from build123d import *

# Parameters (mm, degrees)
F0_R     = 136.525
F0_R_2   = 79.375
F1_DEPTH = 50.8
F2_R     = 31.75
F4_R     = 19.05
F5_DEPTH = 38.1


# Not quite as in the source:
# - a fillet or chamfer that OpenCascade refuses, or shapes differently, is made with other operations: its cross-section is extruded or revolved along the edge and cut away or added


with BuildPart() as f1:
    # F0 (on Top) → F1 (new body)
    with BuildSketch(Plane.XY):
        with Locations((0, 2.0348737297)):
            Circle(F0_R)
        with Locations((0, 2.0348737297)):
            Circle(F0_R_2, mode=Mode.SUBTRACT)
    extrude(amount=F1_DEPTH)

    # F2
    f2_edges = [f1.edges().sort_by_distance(p)[0] for p in [
        (-136.525, 2.034874, 0),
    ]]
    fillet(f2_edges, radius=F2_R)

    # F3: fillet of radius 31.75 on 1 edges, made by hand

    # F3_s1 → F3_t2 (revolve, cut)
    with BuildSketch(Plane.XZ.offset(-2.0348737297)):
        with BuildLine():
            ThreePointArc((104.775, 0), (86.5315557516, 11.0280565913), (79.375, 31.1085197333))
            Line((79.375, 31.1085197333), (79.375, 0))
            Line((79.375, 0), (104.775, 0))
        make_face()
    revolve(axis=Axis((0, 2.0348737297, 0), (0, 0, 1)), mode=Mode.SUBTRACT)

    # F4 (on face) → F5 (cut)
    with BuildSketch(Plane.XY.offset(50.8)):
        with BuildLine():
            ThreePointArc((-83.5406207988, -89.6430518351), (-63.4036145785, -91.8975231455), (-52.6271930456, -74.7379660606))
            ThreePointArc((-52.6271930456, -74.7379660606), (-54.2244900151, -67.1021519632), (-58.7485218572, -60.74682739))
            ThreePointArc((-58.7485218572, -60.74682739), (-86.1351193385, -62.3334964102), (-83.5406207988, -89.6430518351))
        make_face()
        with BuildLine():
            ThreePointArc((-58.7485218572, -60.74682739), (-54.2244900151, -67.1021519632), (-52.6271930456, -74.7379660606))
            ThreePointArc((-52.6271930456, -74.7379660606), (-63.4036145785, -91.8975231455), (-83.5406207988, -89.6430518351))
            add(Edge.make_bspline(
                [(-2.8122035096, -125.8770781244), (-17.2926198403, -124.7913924318), (-47.475617869, -121.9892901593), (-71.1455318862, -100.7416006213), (-83.5406207988, -89.6430518351)],
                knots=[0.0299392112, 0.0299392112, 0.0299392112, 0.0299392112, 0.492539633, 1, 1, 1, 1], degree=3))
            ThreePointArc((-2.8122035096, -125.8770781244), (-18.9977495336, -105.6258243369), (0, -87.985793364))
            add(Edge.make_bspline(
                [(0, -87.985793364), (-10.8720074629, -86.6942500904), (-32.9218918222, -84.0821884123), (-50.0558702898, -68.5889761619), (-58.7485218572, -60.74682739)],
                knots=[0, 0, 0, 0, 0.493177557, 1, 1, 1, 1], degree=3))
        make_face()
        with BuildLine():
            ThreePointArc((19.05, -107.035793364), (13.4703841816, -93.5654091824), (0, -87.985793364))
            ThreePointArc((0, -87.985793364), (-18.9977495336, -105.6258243369), (-2.8122035096, -125.8770781244))
            add(Edge.make_bspline(
                [(0, -126.085793364), (-0.9375128174, -126.0165583722), (-1.8750399814, -125.9473430264), (-2.8122035096, -125.8770781244)],
                knots=[0, 0, 0, 0, 0.0299392112, 0.0299392112, 0.0299392112, 0.0299392112], degree=3))
            ThreePointArc((0, -126.085793364), (13.4703841816, -120.5061775457), (19.05, -107.035793364))
        make_face()
        with Locations((74.0118548274, -77.8447389603)):
            Circle(F4_R)
        with BuildLine():
            add(Edge.make_bspline(
                [(78.9350842893, 101.6695168607), (78.0894264406, 102.3824779177), (77.2423258351, 103.0946725571), (76.3952137559, 103.80686703)],
                knots=[0.9690492423, 0.9690492423, 0.9690492423, 0.9690492423, 1, 1, 1, 1], degree=3))
            ThreePointArc((76.3952137559, 103.80686703), (50.1528602496, 99.5766504715), (53.6856126427, 73.2313376017))
            ThreePointArc((53.6856126427, 73.2313376017), (73.7786820966, 71.0869181488), (84.4960042715, 88.2178544998))
            ThreePointArc((84.4960042715, 88.2178544998), (83.0509676958, 95.4957499944), (78.9350842893, 101.6695168607))
        make_face()
        with BuildLine():
            ThreePointArc((84.4960042715, 88.2178544998), (73.7786820966, 71.0869181488), (53.6856126427, 73.2313376017))
            add(Edge.make_bspline(
                [(84.7416844545, 15.995532865), (84.7371406471, 26.5933171928), (83.3814622914, 49.6305752088), (64.2349565752, 64.8357897445), (53.6856126427, 73.2313376017)],
                knots=[0.0840841786, 0.0840841786, 0.0840841786, 0.0840841786, 0.4948689966, 1, 1, 1, 1], degree=3))
            ThreePointArc((84.7416844545, 15.995532865), (103.773764442, 31.641700355), (122.3236967579, 15.4268109984))
            add(Edge.make_bspline(
                [(122.3236967579, 15.4268109984), (120.6881998826, 33.4274356769), (117.5065684963, 68.2125390548), (91.7120360038, 90.8974664243), (78.9350842893, 101.6695168607)],
                knots=[0, 0, 0, 0, 0.5014176382, 0.9690492423, 0.9690492423, 0.9690492423, 0.9690492423], degree=3))
            ThreePointArc((78.9350842893, 101.6695168607), (83.0509676958, 95.4957499944), (84.4960042715, 88.2178544998))
        make_face()
        with BuildLine():
            ThreePointArc((122.3236967579, 15.4268109984), (103.773764442, 31.641700355), (84.7416844545, 15.995532865))
            add(Edge.make_bspline(
                [(84.6941362488, 9.4655427217), (84.7182599274, 11.6458483909), (84.7426145335, 13.8262560296), (84.7416844545, 15.995532865)],
                knots=[0, 0, 0, 0, 0.0840841786, 0.0840841786, 0.0840841786, 0.0840841786], degree=3))
            ThreePointArc((84.6941362488, 9.4655427217), (105.0550223499, -6.3913539202), (122.5355172038, 12.5938812271))
            ThreePointArc((122.5355172038, 12.5938812271), (122.4824882848, 14.0143000905), (122.3236967579, 15.4268109984))
        make_face()
        with Locations((-106.1858087778, -19.3491019309)):
            Circle(F4_R)
        with Locations((14.8240327835, 111.9937822223)):
            Circle(F4_R)
        with BuildLine():
            add(Edge.make_bspline(
                [(-114.1068806006, 54.731659933), (-114.0705377389, 54.8113823903), (-114.0341951825, 54.8911049607), (-113.9978523202, 54.9708268217)],
                knots=[0, 0, 0, 0, 0.0029673982, 0.0029673982, 0.0029673982, 0.0029673982], degree=3))
            ThreePointArc((-114.1068806006, 54.731659933), (-105.2006835176, 29.8918835009), (-80.0197694208, 37.7821563054))
            add(Edge.make_bspline(
                [(-80.0197694208, 37.7821563054), (-79.3943245384, 41.4243222007), (-78.7675270407, 45.0666971781), (-77.740869501, 48.6034247835)],
                knots=[0, 0, 0, 0, 0.1730413551, 0.1730413551, 0.1730413551, 0.1730413551], degree=3))
            ThreePointArc((-77.740869501, 48.6034247835), (-93.4238298796, 65.7123618791), (-113.9978523202, 54.9708268217))
        make_face()
        with BuildLine():
            add(Edge.make_bspline(
                [(-113.9978523202, 54.9708268217), (-107.6814847314, 68.8264382664), (-95.452579475, 95.5712033941), (-71.1959439676, 106.0972459264), (-59.4868722066, 111.1759600983)],
                knots=[0.0029673982, 0.0029673982, 0.0029673982, 0.0029673982, 0.5186994147, 1, 1, 1, 1], degree=3))
            ThreePointArc((-113.9978523202, 54.9708268217), (-93.4238298796, 65.7123618791), (-77.740869501, 48.6034247835))
            add(Edge.make_bspline(
                [(-77.740869501, 48.6034247835), (-76.0045089103, 54.5850050058), (-70.5050739876, 65.4294674019), (-53.8065169404, 73.305008588), (-47.9266097256, 75.67092688)],
                knots=[0.1730413551, 0.1730413551, 0.1730413551, 0.1730413551, 0.4657019337, 0.7318600546, 0.7318600546, 0.7318600546, 0.7318600546], degree=3))
            ThreePointArc((-47.9266097256, 75.67092688), (-68.2199127162, 88.6980268466), (-59.4868722066, 111.1759600983))
        make_face()
        with BuildLine():
            ThreePointArc((-31.0558846712, 94.5958644152), (-40.5091485737, 111.0520230275), (-59.4868722066, 111.1759600983))
            ThreePointArc((-59.4868722066, 111.1759600983), (-68.2199127162, 88.6980268466), (-47.9266097256, 75.67092688))
            add(Edge.make_bspline(
                [(-47.9266097256, 75.67092688), (-43.5392758956, 77.4362733357), (-40.3063077929, 78.4304649494), (-40.1444315528, 78.3578857303)],
                knots=[0.7318600546, 0.7318600546, 0.7318600546, 0.7318600546, 0.9304557952, 0.9304557952, 0.9304557952, 0.9304557952], degree=3))
            ThreePointArc((-40.1444315528, 78.3578857303), (-33.4825850303, 85.29164983), (-31.0558846712, 94.5958644152))
        make_face()
    extrude(amount=-F5_DEPTH, mode=Mode.SUBTRACT)


solid = f1.part
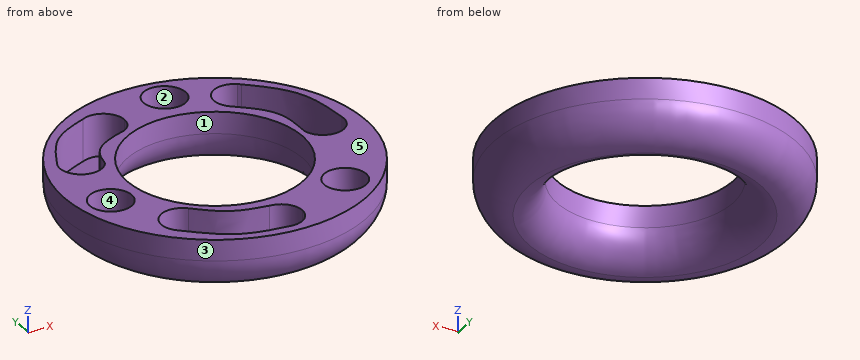
Design review of the part built by this model. Coordinates are the model's own, in mm. Face numbers are marked on the shaded views. A direction names the side the tool comes from. Give positions to 0.01 mm unless a question says otherwise; leave off trailing zeros. Order: outer loops, then holes, each group sorted by start corner. A loop starts at its lowest first (then second) coordinate and runs counter-clockwise, first axis right, second up. Notation, with made-up numbers: (-18.75, -38) - (10.25, -38) arc R18 cw to (10.25, -30) - close; hole circle Ø7 at (52.5, 29). An arc over 180 degrees is marked (long way). Use CSV: the item, a comma, the result in double quotes. Start each with the question number.
Q1. Machinability: for the marked faces 1 and 2, which of the approach directions +Z, -Z, +X, -X, +Y, -Y give a long, thin tool a straight path to every point of the face, cutting with its end or side? Answer none if there is none.
Q2. For P1, Ø1.5, axis at y = -48.5, z = 32, coming from the +X side; P2, Ø12, axis at x = -77, z = 41.5, coming from the -Y side; P3, Ø11.5, axis at x = -99.5, y = -28, coming from the +Z side, all flat-tipped, find the tip position at first contact; note any pin that passes through.
Q3. For line 1 (Y direction, x = -64.5, z = 16); line 2 (X direction, y = 3.5, z = 25); line 3 (Y direction, x = -92.5, z = 30.5), list the stretches that pass through material, from the lowest coordinate up.
Q4. Take a section at A-A (z = 9). State the section outline as (x, y) points.
Q5. Take a section at B-B (z = 24.5). Count the separate pieces of the cut face and the enclosed holes in it, and give its area (3 significant figures).
Q6. Draft analysis for pull direction X (two halves, no side actions). For the marked faces 3, 4 and 5, state which applies: pulls with the +X half, pulls with the -X half, needs draft (parallel to the pull), parting line crosses it, or undercut.
Calculated:
1,face 1,"+Z, -Z"
1,face 2,"+Z"
2,P1,"stops at x = 127.12"
2,P2,"stops at y = -114.58"
2,P3,"stops at z = 12.7"
3,line 1,"y = -113.53 to -105.85, -57.09 to -50.52, 54.59 to 67.13, 108.99 to 117.6"
3,line 2,"x = -135.79 to -79.95, 79.95 to 86.75, 120.22 to 135.79"
3,line 3,"y = -98.34 to -32.6, -6.1 to 28.37, 91.46 to 102.41"
4,outline,"circle Ø253.84 at (0, 2.03); hole circle Ø176.67 at (0, 2.03)"
5,separate pieces,"1"
5,enclosed holes,"7"
5,area,"21,900 mm²"
6,face 3,"parting line crosses it"
6,face 4,"undercut"
6,face 5,"needs draft"
